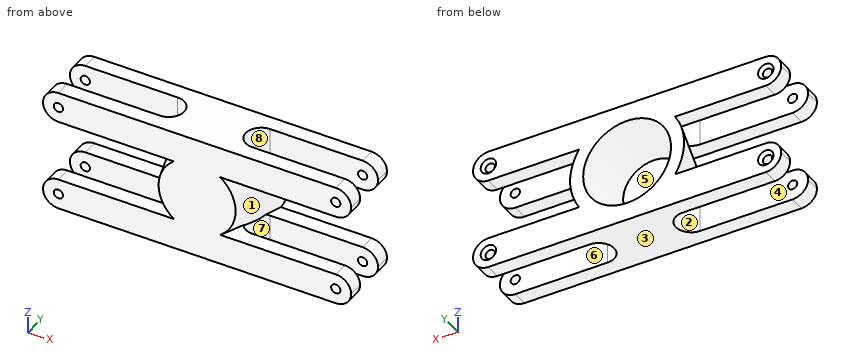
from build123d import *

# Parameters (mm, degrees)
BOSS_EXTRU_1_DEPTH        = 10
ESQUISSE9_R               = 1.5
ENL_V_MAT_EXTRU_1_DEPTH   = 51.249378106
ESQUISSE4_R               = 12.5
ESQUISSE3_R               = 18.5
SYM_TRIE3_COPY_1_DEPTH    = 10
SYM_TRIE3_COPY_2_SKETCH_R = 1.5
SYM_TRIE3_COPY_2_DEPTH    = 51.249378106
CHANFREIN1_SIZE           = 1
BOSS_EXTRU_2_DEPTH        = 10


with BuildPart() as part:
    # Esquisse1 → Boss.-Extru.1 (new body)
    with BuildSketch(Plane.XY):
        with BuildLine():
            Line((0, 0), (35, 0))
            Line((35, 0), (45, 0))
            Line((45, 0), (45, -20))
            Line((45, -20), (35, -20))
            Line((35, -20), (0, -20))
            Line((0, -20), (0, -15))
            Line((0, -15), (35, -15))
            ThreePointArc((35, -15), (40, -10), (35, -5))
            Line((35, -5), (0, -5))
            Line((0, -5), (0, 0))
        make_face()
    boss_extru_1 = extrude(amount=BOSS_EXTRU_1_DEPTH)

    # Esquisse9 → Enlèv. mat.-Extru.1 (cut, symmetric)
    with BuildSketch(Plane(origin=(0, 0, 0), x_dir=(1, 0, 0), z_dir=(0, 1, 0))):
        with BuildLine():
            ThreePointArc((0, -5), (1.464466094, -1.464466094), (5, 0))
            Line((5, 0), (0, 0))
            Line((0, 0), (0, -5))
        make_face()
        with BuildLine():
            ThreePointArc((5, -10), (1.464466094, -8.535533906), (0, -5))
            Line((0, -5), (0, -10))
            Line((0, -10), (5, -10))
        make_face()
        with Locations(Location((5, -5, 0), (0, 0, 270))):
            Circle(ESQUISSE9_R)
    enl_v_mat_extru_1 = extrude(amount=ENL_V_MAT_EXTRU_1_DEPTH, both=True, mode=Mode.SUBTRACT)

    # Esquisse4 → Lissage2 section 0
    with BuildSketch(Plane.XZ.offset(20)):
        with Locations((50, 20)):
            Circle(ESQUISSE4_R)
    # Esquisse3 → Lissage2 section 1
    with BuildSketch(Plane(origin=(0, 0, 0), x_dir=(1, 0, 0), z_dir=(0, 1, 0))):
        with Locations((50, -20)):
            Circle(ESQUISSE3_R)
    loft()

    # Symétrie2: Boss.-Extru.1, Enlèv. mat.-Extru.1 across plane
    add(boss_extru_1.mirror(Plane.XY.offset(20)))
    add(enl_v_mat_extru_1.mirror(Plane.XY.offset(20)), mode=Mode.SUBTRACT)

    # Symétrie3: Boss.-Extru.1, Enlèv. mat.-Extru.1 across plane
    add(boss_extru_1.mirror(Plane(origin=(50, 0, 0), x_dir=(0, 0, 1), z_dir=(1, 0, 0))))
    add(enl_v_mat_extru_1.mirror(Plane(origin=(50, 0, 0), x_dir=(0, 0, 1), z_dir=(1, 0, 0))), mode=Mode.SUBTRACT)

    # Symétrie3 copy 1 sketch → Symétrie3 copy 1 (add)
    with BuildSketch(Plane(origin=(100, 0, 40), x_dir=(-1, 0, 0), z_dir=(0, 0, -1))):
        with BuildLine():
            Line((0, 0), (35, 0))
            Line((35, 0), (45, 0))
            Line((45, 0), (45, -20))
            Line((45, -20), (35, -20))
            Line((35, -20), (0, -20))
            Line((0, -20), (0, -15))
            Line((0, -15), (35, -15))
            ThreePointArc((35, -15), (40, -10), (35, -5))
            Line((35, -5), (0, -5))
            Line((0, -5), (0, 0))
        make_face()
    extrude(amount=SYM_TRIE3_COPY_1_DEPTH)

    # Symétrie3 copy 2 sketch → Symétrie3 copy 2 (cut, symmetric)
    with BuildSketch(Plane(origin=(100, 0, 40), x_dir=(-1, 0, 0), z_dir=(0, 1, 0))):
        with BuildLine():
            ThreePointArc((0, -5), (1.464466094, -1.464466094), (5, 0))
            Line((5, 0), (0, 0))
            Line((0, 0), (0, -5))
        make_face()
        with BuildLine():
            ThreePointArc((5, -10), (1.464466094, -8.535533906), (0, -5))
            Line((0, -5), (0, -10))
            Line((0, -10), (5, -10))
        make_face()
        with Locations(Location((5, -5, 0), (0, 0, 270))):
            Circle(SYM_TRIE3_COPY_2_SKETCH_R)
    extrude(amount=SYM_TRIE3_COPY_2_DEPTH, both=True, mode=Mode.SUBTRACT)

    # Chanfrein1
    chanfrein1_edges = [part.edges().sort_by_distance(p)[0] for p in [
        (5, 0, 36.5),
        (95, 0, 36.5),
        (95, 0, 3.5),
        (5, 0, 3.5),
    ]]
    chamfer(chanfrein1_edges, length=CHANFREIN1_SIZE)


with BuildPart() as boss_extru_2_tool:
    # Esquisse10 → Boss.-Extru.2 (new body)
    with BuildSketch(Plane.ZY.offset(-55)):
        with BuildLine():
            Line((31.456439237, -20), (40, -20))
            Line((40, -20), (40, 0))
            Line((40, 0), (37.811513131, 0))
            add(Edge.make_bspline(
                [(37.811513131, 0), (36.770961966, -3.339421755), (35.724642409, -6.676958136), (33.611133104, -13.345209566), (32.544444679, -16.67608847), (31.456439237, -20)],
                knots=[0, 0, 0, 0, 0.5, 0.5, 1, 1, 1, 1], degree=3))
        make_face()
        with BuildLine():
            Line((0, -20), (8.543560763, -20))
            add(Edge.make_bspline(
                [(8.543560763, -20), (7.455555321, -16.67608847), (6.388866896, -13.345209566), (4.275357591, -6.676958136), (3.229038034, -3.339421755), (2.188486869, 0)],
                knots=[0, 0, 0, 0, 0.5, 0.5, 1, 1, 1, 1], degree=3))
            Line((2.188486869, 0), (0, 0))
            Line((0, 0), (0, -20))
        make_face()
    extrude(amount=BOSS_EXTRU_2_DEPTH)


with BuildPart() as part_1:
    add(part.part)


with BuildPart() as part_2:
    # Boss.-Extru.2: joined with boss_extru_2_tool
    add(part_1.part.fuse(boss_extru_2_tool.part, tol=0.00001))

    # Enlèvement de matière-Lissage1: read off the stored shape, not the designer's step
    # Enlèvement de matière-Lissage1: loft between two sections, ruled curve by curve
    enl_vement_de_mati_re_lissage1_from = [
        Edge.make_bspline([(40.172449115, -15, 18.150880317), (36.47420975, -15, 37.805982088), (56.12931152, -15, 41.504221453), (59.827550885, -15, 21.849119683), (63.52579025, -15, 2.194017912), (43.87068848, -15, -1.504221453), (40.172449115, -15, 18.150880317)], [0, 0, 0, 0, 0.5, 0.5, 0.5, 1, 1, 1, 1], 3, [1, 0.333333333, 0.333333333, 1, 0.333333333, 0.333333333, 1]),
    ]
    enl_vement_de_mati_re_lissage1_to = [
        Edge.make_bspline([(35.80353412, 0, 21.234040725), (38.271615569, 0, 49.626972485), (66.66454733, 0, 47.158891036), (64.19646588, 0, 18.765959275), (61.728384431, 0, -9.626972485), (33.33545267, 0, -7.158891036), (35.80353412, 0, 21.234040725)], [0, 0, 0, 0, 0.5, 0.5, 0.5, 1, 1, 1, 1], 3, [1, 0.333333333, 0.333333333, 1, 0.333333333, 0.333333333, 1]),
    ]
    enl_vement_de_mati_re_lissage1 = Solid(Shell([*[Face.make_surface_from_curves(enl_vement_de_mati_re_lissage1_from[k], enl_vement_de_mati_re_lissage1_to[k]) for k in range(1)], Face(Wire(enl_vement_de_mati_re_lissage1_from)), Face(Wire(enl_vement_de_mati_re_lissage1_to))]))
    add(enl_vement_de_mati_re_lissage1, mode=Mode.SUBTRACT)


solid = part_2.part
Design review of the part built by this model. Coordinates are the model's own, in mm. Face numbers are marked on the shaded views. A direction names the side the tool comes from. Round coordinates to 2 decimals unless told otherwise and drop trailing zeros. Loops run counter-clockwise (first coordinate to the right, second up) from the corner with the lowest first, then second, coordinate; pieces in that order, holes last. Notation, with made-up numbers: M -37.75,29 L -6.75,29 A18 ccw -6.75,61 Z; hole C 21,72.5 d10. An arc over 180 degrees is marked long. Answer as a JSON object with one key per item and string values.
Item 1: Clearance check with flat-ended pins moving along their axes: P1, Ø4, axis at x = 95, z = 35, coming from the +Y side; P2, Ø2, axis at y = -16, z = 23, coming from the +X side. State where each tip first meets the part, or that it passes through.
Answer sheet:
{"P1": "stops at y = -0.5", "P2": "stops at x = 63.73"}
Item 2: Machinability: for the marked faces 4, 5, 6, 7 and 8, which of the approach directions +Z, -Z, +X, -X, +Y, -Y give a long, thin tool a straight path to every point of the face, cutting with its end or side? Answer none if there is none.
Answer sheet:
{"face 4": "+Z, -Z, -X", "face 5": "+Y", "face 6": "+Z, -Z, +X", "face 7": "-Z, +X", "face 8": "+Z, +X"}
Item 3: We need section A-A on x = 76. Give the boundary of the cut face in (y, z), and give its area (3 significant figures).
Answer sheet:
{"outline": "M -20,0 L -15,0 L -15,10 L -20,10 Z; M -20,30 L -15,30 L -15,40 L -20,40 Z; M -5,0 L 0,0 L 0,10 L -5,10 Z; M -5,30 L 0,30 L 0,40 L -5,40 Z", "area": "200 mm^2"}
Item 4: The part is to be moulded in two halves that separate along Z. For the marked faces 1, 2 and 3, say which applies: pulls with the +Z half, pulls with the -Z half, needs draft (parallel to the pull), parting line crosses it, or undercut.
Answer sheet:
{"face 1": "undercut", "face 2": "needs draft", "face 3": "pulls with the -Z half"}
Item 5: Wall thickness on L1, parallel to Z at x = 95, y = -16.9; L2, parallel to X at y = -18.35, z = 5; L3, parallel to Y at x = 27, z = 9: over which ranges is each line inside the solid? List them lowest first. Write a range as from..to.
Answer sheet:
{"L1": "z = 0..3.5, 6.5..10, 30..33.5, 36.5..40", "L2": "x = 0..3.5, 6.5..93.5, 96.5..100", "L3": "y = -20..-15, -5..0"}
